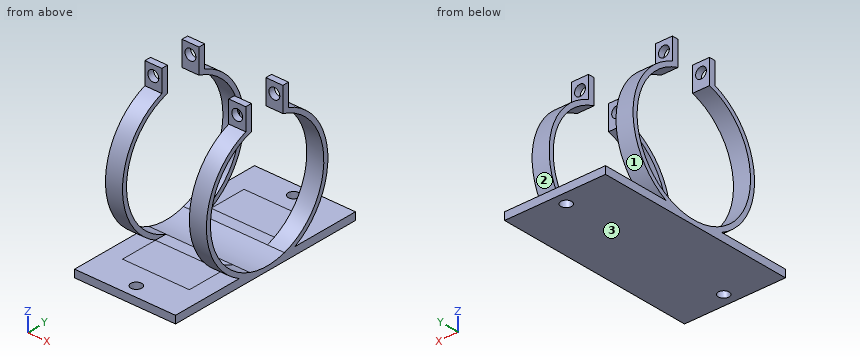
```python
from build123d import *

# Parameters (mm, degrees)
SKETCH1_W           = 40
SKETCH1_H           = 80
SKETCH1_R           = 2.15
BOSS_EXTRUDE1_DEPTH = 3
BOSS_EXTRUDE2_DEPTH = 40
SKETCH3_R           = 25.2
CUT_EXTRUDE1_DEPTH  = 40
CUT_EXTRUDE2_REACH  = 110.225
SKETCH5_W           = 26.5
SKETCH5_H           = 54
SKETCH6_R           = 2.15
CUT_EXTRUDE3_DEPTH  = 89.527071115
SKETCH7_R           = 2.15
CUT_EXTRUDE4_DEPTH  = 89.527071115


with BuildPart() as part:
    # Sketch1 → Boss-Extrude1 (new body)
    with BuildSketch(Plane.XY):
        with Locations((20, 40)):
            Rectangle(SKETCH1_W, SKETCH1_H)
        with Locations((20, 75)):
            Circle(SKETCH1_R, mode=Mode.SUBTRACT)
        with Locations((20, 5)):
            Circle(SKETCH1_R, mode=Mode.SUBTRACT)
    extrude(amount=BOSS_EXTRUDE1_DEPTH)

    # Sketch2 → Boss-Extrude2 (add)
    with BuildSketch(Plane.ZY):
        with BuildLine():
            Line((51.208263052, 47.742845654), (60.931919228, 47.742845654))
            Line((60.931919228, 47.742845654), (60.931919228, 50.242845654))
            Line((60.931919228, 50.242845654), (52.273503912, 50.242845654))
            ThreePointArc((52.273503912, 50.242845654), (0, 40.742845654), (52.273503912, 31.242845654))
            Line((52.273503912, 31.242845654), (60.931919228, 31.242845654))
            Line((60.931919228, 31.242845654), (60.931919228, 33.742845654))
            Line((60.931919228, 33.742845654), (51.208263052, 33.742845654))
            ThreePointArc((51.208263052, 33.742845654), (1.8, 40.742845654), (51.208263052, 47.742845654))
        make_face()
    extrude(amount=-BOSS_EXTRUDE2_DEPTH)

    # Sketch3 → Cut-Extrude1 (cut)
    with BuildSketch(Plane.ZY):
        with Locations((27, 40.742845654)):
            Circle(SKETCH3_R)
    extrude(amount=-CUT_EXTRUDE1_DEPTH, mode=Mode.SUBTRACT)

    # Cut-Extrude2: up to this face of the body (flat: up to its plane)
    cut_extrude2_end = Plane(part.part.faces().sort_by_distance((20, 66.440507587, 3))[0])
    # Sketch5 → Cut-Extrude2 (cut, up to the picked face)
    with BuildSketch(Plane.XY.offset(60.931919228), mode=Mode.PRIVATE) as cut_extrude2_sk1:
        with Locations((20, 40.742845654)):
            Rectangle(SKETCH5_W, SKETCH5_H)
    cut_extrude2_tool1 = split(extrude(cut_extrude2_sk1.sketch, amount=-CUT_EXTRUDE2_REACH, mode=Mode.PRIVATE), bisect_by=cut_extrude2_end, keep=Keep.BOTH, mode=Mode.PRIVATE)
    add(cut_extrude2_tool1.solids().sort_by(Axis((20, 40.742846, 60.931919), (0, 0, -1)))[0], mode=Mode.SUBTRACT)

    # Sketch6 → Cut-Extrude3 (cut, through all)
    with BuildSketch(Plane(origin=(0, 50.242845654, 0), x_dir=(1, 0, 0), z_dir=(0, 1, 0))):
        with Locations(Location((3.375, -56.940793842, 0), (0, 0, 270))):
            Circle(SKETCH6_R)
        with Locations((21.625, -56.940793842)):
            Circle(SKETCH6_R)
    extrude(amount=-CUT_EXTRUDE3_DEPTH, mode=Mode.SUBTRACT)

    # Sketch7 → Cut-Extrude4 (cut, through all)
    with BuildSketch(Plane(origin=(0, 50.242845654, 0), x_dir=(1, 0, 0), z_dir=(0, 1, 0))):
        with Locations(Location((36.625, -56.75422316, 0), (0, 0, 270))):
            Circle(SKETCH7_R)
    extrude(amount=-CUT_EXTRUDE4_DEPTH, mode=Mode.SUBTRACT)


solid = part.part
```
Could you check a few things on this model? Use its own coordinates, in mm. Face numbers are marked on the shaded views. Coordinates: 2 decimals unless noted, no trailing zeros. Write each loop counter-clockwise with the first axis right and the second up, starting at its lowest first coordinate (ties: lowest second). Pieces come first, ordered by that corner, then holes. Notation, with made-up numbers: (19.25, 78) -> (36.25, 78) arc R29 cw to (36.25, 114) -> close; hole circle Ø1 at (69.5, 48). An arc over 180 degrees is marked (long way). Return JSON: item names as keys, results as strings.
(1) Imagine slicing it at B-B, the plane y = 5. Please give me the cut outline in (x, z).
Numbers:
{"outline": "(0, 0) -> (17.85, 0) -> (17.85, 3) -> (0, 3) -> close; (22.15, 0) -> (40, 0) -> (40, 3) -> (22.15, 3) -> close"}
(2) We'd pull the mould along Z, two halves only. Please class the marked faces 1, 2 and 3: +Z half, -Z half, draft (parallel to the pull), parting line (faces both ways), or undercut.
Numbers:
{"face 1": "undercut", "face 2": "undercut", "face 3": "-Z half"}
(3) I need wall thicknesses on L1, parallel to Y at x = 20, z = 1.45; L2, parallel to Z at x = 3.5, y = 21.5; L3, parallel to Z at x = 37, y = 63. Which ranges of each line are inside material? Lowest first, please.
Numbers:
{"L1": "y = 0 to 2.85, 7.15 to 72.85, 77.15 to 80", "L2": "z = 0 to 3, 8.06 to 10.73, 43.27 to 45.94", "L3": "z = 0 to 3, 11.72 to 15.18, 38.82 to 42.28"}
(4) Imagine slicing it at C-C, the plane z = 32. Please give me the cut outline in (x, y).
Numbers:
{"outline": "(0, 14.21) -> (6.75, 14.21) -> (6.75, 16.04) -> (0, 16.04) -> close; (0, 65.44) -> (6.75, 65.44) -> (6.75, 67.28) -> (0, 67.28) -> close; (33.25, 14.21) -> (40, 14.21) -> (40, 16.04) -> (33.25, 16.04) -> close; (33.25, 65.44) -> (40, 65.44) -> (40, 67.28) -> (33.25, 67.28) -> close"}
(5) Imagine slicing it at A-A, the plane x = 20. Please give me the cut outline in (y, z).
Numbers:
{"outline": "(0, 0) -> (2.85, 0) -> (2.85, 3) -> (0, 3) -> close; (7.15, 0) -> (72.85, 0) -> (72.85, 3) -> (48.43, 3) arc R25.2 cw to (33.06, 3) -> (7.15, 3) -> close; (77.15, 0) -> (80, 0) -> (80, 3) -> (77.15, 3) -> close"}
(6) Imagine slicing it at D-D, the plane x = 24.5. Please give me the cut outline in (y, z), then the cut area to 3 significant figures.
Numbers:
{"outline": "(0, 0) -> (80, 0) -> (80, 3) -> (48.43, 3) arc R25.2 cw to (33.06, 3) -> (0, 3) -> close", "area": "228 mm2"}
(7) I'm going to push flat-ended pins straight in: pin 1 (3 mm diameter, centred on x = 7.5, y = 22, fed in from +Z); pin 2 (3.5 mm diameter, centred on x = 3.5, z = 57.5, fed in from -Y); pin 3 (5 mm diameter, centred on x = 20, y = 5, fed in from +Z); pin 4 (16 mm diameter, centred on y = 59, z = 20.5, fed in from -X). Where does each tip first touch, or does it pass through?
Numbers:
{"pin 1": "stops at z = 47.61", "pin 2": "stops at y = 31.24", "pin 3": "stops at z = 3", "pin 4": "stops at x = 0"}
